Geometry: final body of the model. Coordinates: model frame, mm. A direction names the side the tool comes from. Round coordinates to 2 decimals unless told otherwise and drop trailing zeros. Loops run counter-clockwise (first coordinate to the right, second up) from the corner with the lowest first, then second, coordinate; pieces in that order, holes last. Notation, with made-up numbers: M 59.25,52 L 76.25,52 A29 cw 76.25,76 Z; hole C -31,54.25 d3. An arc over 180 degrees is marked long. Answer as a JSON object with one key per item and string values.
from build123d import *

# Parameters (mm, degrees)
SKETCH1_W            = 254
SKETCH1_H            = 127
BOSS_EXTRUDE1_DEPTH  = 6.35
SKETCH3_R            = 2.54
CUT_EXTRUDE3_DEPTH   = 25.4
LPATTERN1_COUNT      = 4
LPATTERN1_PITCH      = 20.32
SKETCH3_7_R          = 2.54
CUT_EXTRUDE4_DEPTH   = 25.4
LPATTERN2_COUNT      = 7
LPATTERN2_PITCH      = 14.9999954
LPATTERN2_COUNT_DIR2 = 5
LPATTERN2_PITCH_DIR2 = 14.9999954
SKETCH3_8_R          = 32.004
SKETCH3_8_R_2        = 2.54
SKETCH3_8_R_3        = 2.0574
SKETCH3_8_W          = 12.192
SKETCH3_8_H          = 21.336
CUT_EXTRUDE5_DEPTH   = 25.4


with BuildPart() as part:
    # Sketch1 → Boss-Extrude1 (new body)
    with BuildSketch(Plane(origin=(0, 0, 0), x_dir=(1, 0, 0), z_dir=(0, 1, 0))):
        with Locations((-62.014339623, -15.479622642)):
            Rectangle(SKETCH1_W, SKETCH1_H)
    extrude(amount=BOSS_EXTRUDE1_DEPTH)

    # Sketch3 → Cut-Extrude3 (cut)
    with BuildSketch(Plane(origin=(0, 6.35, 0), x_dir=(1, 0, 0), z_dir=(0, 1, 0))):
        with Locations((57.365660377, 15.000377358)):
            Circle(SKETCH3_R)
    cut_extrude3 = extrude(amount=-CUT_EXTRUDE3_DEPTH, mode=Mode.SUBTRACT)

    # LPattern1: Cut-Extrude3 ×4
    with Locations(*[(0, 0, i * LPATTERN1_PITCH) for i in range(1, LPATTERN1_COUNT)]):
        add(cut_extrude3, mode=Mode.SUBTRACT)

    # Sketch3<7> → Cut-Extrude4 (cut)
    with BuildSketch(Plane(origin=(0, 6.35, 0), x_dir=(1, 0, 0), z_dir=(0, 1, 0))):
        with Locations((-106.972339623, 14.492377358)):
            Circle(SKETCH3_7_R)
    cut_extrude4 = extrude(amount=-CUT_EXTRUDE4_DEPTH, mode=Mode.SUBTRACT)

    # LPattern2: Cut-Extrude4 7 × 5
    with Locations(*[(i * LPATTERN2_PITCH, 0, j * LPATTERN2_PITCH_DIR2) for i in range(LPATTERN2_COUNT) for j in range(LPATTERN2_COUNT_DIR2) if (i, j) != (0, 0)]):
        add(cut_extrude4, mode=Mode.SUBTRACT)

    # Sketch3<8> → Cut-Extrude5 (cut)
    with BuildSketch(Plane(origin=(0, 6.35, 0), x_dir=(1, 0, 0), z_dir=(0, 1, 0))):
        with Locations((-145.834339623, -15.479622642)):
            Circle(SKETCH3_8_R)
        with Locations((21.805660377, -15.479622642)):
            Circle(SKETCH3_8_R)
        with Locations((-106.972339623, 14.492377358)):
            Circle(SKETCH3_8_R_2)
        with Locations((-172.504339623, -42.149622642)):
            Circle(SKETCH3_8_R_3)
        with Locations((57.365660377, 15.000377358)):
            Circle(SKETCH3_8_R_2)
        with Locations((-164.122339623, 29.732377358)):
            Circle(SKETCH3_8_R_2)
        with Locations((-119.164339623, -42.149622642)):
            Circle(SKETCH3_8_R_3)
        with Locations((-172.504339623, 11.190377358)):
            Circle(SKETCH3_8_R_3)
        with Locations((-119.164339623, 11.190377358)):
            Circle(SKETCH3_8_R_3)
        with Locations((-4.864339623, -42.149622642)):
            Circle(SKETCH3_8_R_3)
        with Locations((48.475660377, -42.149622642)):
            Circle(SKETCH3_8_R_3)
        with Locations((-4.864339623, 11.190377358)):
            Circle(SKETCH3_8_R_3)
        with Locations((48.475660377, 11.190377358)):
            Circle(SKETCH3_8_R_3)
        with Locations((-175.298339623, 29.732377358)):
            Rectangle(SKETCH3_8_W, SKETCH3_8_H)
    extrude(amount=-CUT_EXTRUDE5_DEPTH, mode=Mode.SUBTRACT)


solid = part.part
1) Pull-direction query (Z, two-part tool) for faces 3 (the flat face through (-64, 3, -48.02)), 4 (the cylindrical face through (-78.99, 3.22, 32.05)), 5 (the flat face through (-36, 6.35, 15)); classes: +Z half, -Z half, draft (parallel to the pull), parting line (faces both ways), or undercut.
Results:
{"face 3": "-Z half", "face 4": "undercut", "face 5": "draft"}
2) Ray query, line 1 (Z direction, x = -48, y = 0.5); line 2 (X direction, y = 4, z = 23.5); line 3 (X direction, y = 4.5, z = 7). Return the intervals inside material, ascending.
Results:
{"line 1": "-48.02 to -16.82, -12.17 to -1.82, 2.83 to 13.18, 17.83 to 28.18, 32.83 to 43.18, 47.83 to 78.98", "line 2": "-189.01 to -176.82, -114.85 to -9.18, 52.79 to 56, 58.73 to 64.99", "line 3": "-189.01 to -176.69, -114.97 to -9.05, 52.67 to 55.46, 59.27 to 64.99"}
3) Section query B-B (z = -6). Return the cut outline in (x, y).
Results:
{"outline": "M -189.01,0 L -169.56,0 L -169.56,6.35 L -189.01,6.35 Z; M -122.11,0 L -1.92,0 L -1.92,6.35 L -122.11,6.35 Z; M 45.53,0 L 64.99,0 L 64.99,6.35 L 45.53,6.35 Z"}
4) Pin query (flat end, axial travel): P1, Ø3, axis at x = -31.97, z = -14.49, coming from the +Y side. Return the tip coordinate at first contact, or that it passes through.
Results:
{"P1": "through"}
5) Section query A-A (x = 36). Return the cut outline in (y, z), and give its area (3 significant figures).
Results:
{"outline": "M 0,-48.02 L 6.35,-48.02 L 6.35,-13.2 L 0,-13.2 Z; M 0,44.16 L 6.35,44.16 L 6.35,78.98 L 0,78.98 Z", "area": "442 mm2"}
6) Reachability of faces 1 (the flat face through (-175, 3, -40.4)), 2 (the flat face through (-64, 3, 78.98)) from +Z, -Z, +X, -X, +Y, -Y: full face, straight path, thin tool, end or side. Return the list, or none.
Results:
{"face 1": "+Y, -Y", "face 2": "+Z, +X, -X, +Y, -Y"}
7) Section query C-C (x = -153.5). Return the cut outline in (y, z).
Results:
{"outline": "M 0,-48.02 L 6.35,-48.02 L 6.35,-15.59 L 0,-15.59 Z; M 0,46.55 L 6.35,46.55 L 6.35,78.98 L 0,78.98 Z"}
8) Section query D-D (y = 4.25). Count the separate pieces of the cut face and the enclosed holes in it, and give its area (3 significant figures).
Results:
{"separate pieces": "1", "enclosed holes": "51", "area": "24,600 mm2"}
